For this review, take the finished solid that the model builds, in its own axes (mm). Face numbers are marked on the shaded views. A direction names the side the tool comes from. Coordinates: 2 decimals unless noted, no trailing zeros. Order: outer loops, then holes, each group sorted by start corner. A loop starts at its lowest first (then second) coordinate and runs counter-clockwise, first axis right, second up. Notation, with made-up numbers: (-22, -26) -> (14, -26) arc R32 cw to (14, 3) -> close; hole circle Ø10 at (69.25, 55). An arc over 180 degrees is marked (long way). Return JSON: item names as keys, results as strings. Group by question number.
Item 1: Machinability: for the marked faces 4 and 5, which of the approach directions +Z, -Z, +X, -X, +Y, -Y give a long, thin tool a straight path to every point of the face, cutting with its end or side? Answer none if there is none.
Item 2: Take a section at B-B (z = -1.5). Write out the cut boundary in (x, y), then the cut area to 3 significant figures.
Item 3: Insertion check: pin 1 (0.5 mm diameter, centred on x = 1.5, z = -0.5, fed in from +Y); pin 2 (2 mm diameter, centred on x = -1.5, z = -2, fed in from -Y); pin 3 (0.8 mm diameter, centred on x = -1, z = -0.5, fed in from +Y). Each pin has a flat end and moves straight along its axis. Give the tip position at first contact, or say it passes through.
Item 4: Draft analysis for pull direction Y (two halves, no side actions). For the marked faces 1, 2 and 3, state which applies: +Y half, -Y half, draft (parallel to the pull), parting line (faces both ways), or undercut.
Item 5: For line 1 along X through (y, z) = (-1.5, -0.5); line 2 along Y through (x, z) = (0, -0.75); line 3 along X through (y, z) = (1.5, -0.75), list the stretches that pass through material, from the lowest coordinate up.
Item 6: Take a section at A-A (z = -4.5). Write out the cut boundary in (x, y), then the cut area to 3 significant figures.
```python
from build123d import *

# Parameters (mm, degrees)
BOSS_EXTRUDE3_START = -1
SKETCH1_R           = 3
BOSS_EXTRUDE3_DEPTH = 1.4
DOME1_FACE_RADIUS   = 3
DOME1_HEIGHT        = 1
SKETCH4_R           = 1.5
BOSS_EXTRUDE4_DEPTH = 4
SKETCH5_W           = 2.25
SKETCH5_H           = 0.5
SKETCH5_W_2         = 0.5
SKETCH5_H_2         = 2.25
CUT_EXTRUDE1_DEPTH  = 1


with BuildPart() as part:
    # Sketch1 → Boss-Extrude3 (new body)
    with BuildSketch(Plane.XY.offset(BOSS_EXTRUDE3_START)):
        Circle(SKETCH1_R)
    extrude(amount=-BOSS_EXTRUDE3_DEPTH)

    # Dome1: an elliptical dome of height H over a round flat face of radius A is half a spheroid: the quarter ellipse of half axes A and H revolved about the face's axis
    with BuildSketch(Plane((0, 0, -1), x_dir=(0, 1, 0), z_dir=(1, 0, 0)), mode=Mode.PRIVATE) as dome1_quarter:
        Ellipse(DOME1_FACE_RADIUS, DOME1_HEIGHT)
        Rectangle(DOME1_FACE_RADIUS, DOME1_HEIGHT, align=(Align.MIN, Align.MIN), mode=Mode.INTERSECT)
    revolve(dome1_quarter.sketch, axis=Axis((0, 0, -1), (0, 0, 1)))

    # Sketch4 → Boss-Extrude4 (add)
    with BuildSketch(Plane(origin=(0, 0, -2.4), x_dir=(-1, 0, 0), z_dir=(0, 0, -1))):
        with Locations(Location((0, 0, 0), (0, 0, 180))):
            Circle(SKETCH4_R)
    extrude(amount=BOSS_EXTRUDE4_DEPTH)

    # Sketch5 → Cut-Extrude1 (cut)
    with BuildSketch(Plane.XY):
        with Locations((-1.375, 0)):
            Rectangle(SKETCH5_W, SKETCH5_H)
        Rectangle(SKETCH5_W_2, SKETCH5_H)
        with Locations((0, 1.375)):
            Rectangle(SKETCH5_W_2, SKETCH5_H_2)
        with Locations((1.375, 0)):
            Rectangle(SKETCH5_W, SKETCH5_H)
        with Locations((0, -1.375)):
            Rectangle(SKETCH5_W_2, SKETCH5_H_2)
    extrude(amount=-CUT_EXTRUDE1_DEPTH, mode=Mode.SUBTRACT)


solid = part.part
```
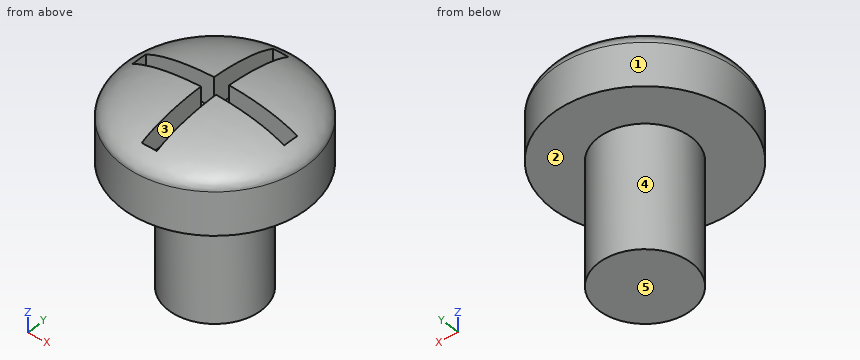
Findings below:
{
 "1": {"face 4": "-Z", "face 5": "-Z, +X, -X, +Y, -Y"},
 "2": {"outline": "circle Ø6 at (0, 0)", "area": "28.3 mm2"},
 "3": {"pin 1": "stops at y = 2.53", "pin 2": "stops at y = -2.96", "pin 3": "stops at y = 2.85"},
 "4": {"face 1": "parting line", "face 2": "draft", "face 3": "undercut"},
 "5": {"line 1": "x = -2.12 to -0.25, 0.25 to 2.12", "line 2": "y = -2.9 to -2.5, 2.5 to 2.9", "line 3": "x = -2.49 to -0.25, 0.25 to 2.49"},
 "6": {"outline": "circle Ø3 at (0, 0)", "area": "7.07 mm2"}
}
